Autodesk Inventor part; units mm, degrees
ref_plane "YZ Plane" through (0, 0, 0) normal (1, 0, 0) x (0, 1, 0)
ref_plane "XZ Plane" through (0, 0, 0) normal (0, 1, 0) x (-1, 0, 0)
ref_plane "XY Plane" through (0, 0, 0) normal (0, 0, 1) x (1, 0, 0)
ref_plane "Arbeitsebene1" through (0, 0, 0) normal (0, 0, 1) x (1, 0, 0)
sketch "Skizze1" plane through (0, 0, 0) normal (0, 0, 1) x (1, 0, 0)
  line L0 (6, 5) -> (6, 20.6772)
  line L1 (25.0752, 5) -> (6, 5)
  line L2 (20.3151, 15.4507) -> (25.0752, 5)
  line L3 (6, 20.6772) -> (20.3151, 15.4507)
  circle A0 centre (28.7957, 2.7835) radius 1.4
  circle A1 centre (22.3001, 17.2899) radius 1.4
  line L4 (32.7967, 0.1099) -> (23.0022, 21.6136)
  arc A2 (30.9766, -2.7191) -> (32.7967, 0.1099) centre (30.9766, -0.7191) ccw
  line L5 (29.8778, -2.7191) -> (30.9766, -2.7191)
  arc A3 (28.0577, -1.5481) -> (29.8778, -2.7191) centre (29.8778, -0.7191) ccw
  line L6 (27.3526, 0) -> (28.0577, -1.5481)
  line L7 (0, 0) -> (27.3526, 0)
  line L8 (0, 0) -> (0, 26)
  line L9 (0, 26) -> (6, 26)
  line L10 (23.0022, 21.6136) -> (18.452, 19.5411)
  line L11 (18.452, 19.5411) -> (34.0518, -14.708)
  line L12 (34.0518, -14.708) -> (38.602, -12.6355)
  line L13 (38.602, -12.6355) -> (23.0022, 21.6136)
  line L14 (23.4977, 22.9382) -> (17.1274, 20.0366)
  line L15 (17.1274, 20.0366) -> (32.7273, -14.2125)
  line L16 (35.3764, -15.2036) -> (38.1065, -13.96)
  line L17 (39.0976, -11.3109) -> (23.4977, 22.9382)
  arc A4 (38.1065, -13.96) -> (39.0976, -11.3109) centre (37.2775, -12.1399) ccw
  arc A5 (32.7273, -14.2125) -> (35.3764, -15.2036) centre (34.5474, -13.3835) ccw
  point P0 (22.6951, 10.2253)
  point P1 (28.0577, -1.5481)
  point P2 (26.2537, 0)
  point P3 (18.9971, 15.9319)
  dimension "d2" = 1
  dimension "d3" = 2
extrude "Extrusion1" add sketch "Skizze1" along normal mid plane 16 contours L15 L3 L2 L1 | L1 L11 L7 L15 | L15 L14 L17 A4 L16 A5 L7 L6 L11 L12 L13 L4 L10 L3 | L2 L11 L10 L4 A2 L5 A3 L6 | A3 L5 A2 L13 L12 L11
properties part number "Gripper_linear_finger_long"
Read the model definition and answer for the solid it produces. Units are mm, in the model's axes. Give positions to 0.01 mm unless a question says otherwise; leave off trailing zeros. Write each loop counter-clockwise with the first axis right and the second up, starting at its lowest first coordinate (ties: lowest second). Pieces come first, ordered by that corner, then holes. Notation, with made-up numbers: (21, -35.5) -> (67, -35.5) arc R25 cw to (67, -10.5) -> close; hole circle Ø5 at (46, -0.5). An arc over 180 degrees is marked (long way). Answer as a JSON object with one key per item and string values.
1) Section B-B on y = 10.5 is taken. Write down the section's boundary in (x, z), then the cut area to 3 significant figures.
Findings below:
{"outline": "(21.47, -8) -> (29.16, -8) -> (29.16, 8) -> (21.47, 8) -> close", "area": "123 mm^2"}
2) Section A-A on z = 0.75 is taken. Write down the section's boundary in (x, y), then the cut area to 3 significant figures.
Findings below:
{"outline": "(17.13, 20.04) -> (32.73, -14.21) arc R2 ccw to (35.38, -15.2) -> (38.11, -13.96) arc R2 ccw to (39.1, -11.31) -> (23.5, 22.94) -> close; hole circle Ø2.8 at (22.3, 17.29); hole circle Ø2.8 at (28.8, 2.78)", "area": "263 mm^2"}
3) Section C-C on x = 26.75 is taken. Write down the section's boundary in (y, z), then the cut area to 3 significant figures.
Findings below:
{"outline": "(-1.09, -8) -> (15.8, -8) -> (15.8, 8) -> (-1.09, 8) -> close", "area": "270 mm^2"}
4) For a pull along Y with two mould halves and no side action, classify faces 1 (the flat face through (31.41, 5.57, -0.11)), 2 (the flat face through (24.82, 3.15, -0.11)), 3 (the cylindrical face through (30.09, 3.32, -0.11)) as pulls with the +Y half, pulls with the -Y half, needs draft (parallel to the pull), parting line crosses it, or undercut.
Findings below:
{"face 1": "pulls with the +Y half", "face 2": "pulls with the -Y half", "face 3": "undercut"}
5) Straight lines are drawn through the part: probe 1 along X at (y, z) = (2, 6.75); probe 2 along Y at (x, z) = (28.5, -7.25); probe 3 along Y at (x, z) = (29.25, 6). For each, find the intervals that lie inside material, in ascending order. Write a range as from..to.
Findings below:
{"probe 1": "x = 25.34..27.64, 29.96..33.03", "probe 2": "y = -4.93..1.42, 4.15..11.96", "probe 3": "y = -6.58..1.46, 4.11..10.31"}
6) Flat-ended cylindrical pins translate along their axes: pin 1 Ø6 at (y, z) = (8.5, -3) entering from -X; pin 2 Ø3.5 at (x, y) = (22.3, 17.29) entering from -Z; pin 3 Ø3 at (x, z) = (36, -4) entering from +Y; pin 4 Ø1.7 at (x, y) = (28.8, 2.78) entering from -Z. Find the tip coordinate at first contact, or state that the pin passes through.
Findings below:
{"pin 1": "stops at x = 21.02", "pin 2": "stops at z = -8", "pin 3": "stops at y = -1.22", "pin 4": "passes through"}
